```python
from build123d import *

# Parameters (mm, degrees)
SKETCH1_W            = 69
SKETCH1_H            = 165
BOSS_EXTRUDE1_DEPTH  = 7
SKETCH3_R            = 2.6
CUT_EXTRUDE2_DEPTH   = 7
SKETCH2_R            = 2.6
CUT_EXTRUDE1_DEPTH   = 7
SKETCH5_W            = 10
SKETCH5_H            = 10
BOSS_EXTRUDE2_DEPTH  = 23.264128691
SKETCH6_R            = 2.25
CUT_EXTRUDE3_DEPTH   = 10
FILLET1_R            = 10
FILLET1_OF_MIRROR1_R = 10
MIRROR2_START        = 123.910418582
MIRROR2_DEPTH        = 2.75
MIRROR2_START_2      = 116.660418582
MIRROR2_2_DEPTH      = 2.7499999
MIRROR2_START_3      = 119.410418482
MIRROR2_3_DEPTH      = 4.5000001
MIRROR2_START_4      = -23.264128691
MIRROR2_4_OUTLINE_R  = 2.25
MIRROR2_4_DEPTH      = 10


with BuildPart() as part:
    # Sketch1 → Boss-Extrude1 (new body)
    with BuildSketch(Plane.XY):
        with Locations((92.160418582, 14.328579343)):
            Rectangle(SKETCH1_W, SKETCH1_H)
    extrude(amount=BOSS_EXTRUDE1_DEPTH)

    # Sketch3 → Cut-Extrude2 (cut)
    with BuildSketch(Plane.XY.offset(7)):
        with Locations((109.883329943, 54.328579343)):
            Circle(SKETCH3_R)
        with Locations((109.883329943, -25.671420657)):
            Circle(SKETCH3_R)
    extrude(amount=-CUT_EXTRUDE2_DEPTH, mode=Mode.SUBTRACT)

    # Sketch2 → Cut-Extrude1 (cut)
    with BuildSketch(Plane.XY.offset(7)):
        with Locations((71.267526747, -59.671420657)):
            Circle(SKETCH2_R)
        with Locations((71.267526747, -15.671420657)):
            Circle(SKETCH2_R)
        with Locations((71.267526747, -7.671420657)):
            Circle(SKETCH2_R)
        with Locations((71.267526747, 36.328579343)):
            Circle(SKETCH2_R)
        with Locations((71.267526747, 44.328579343)):
            Circle(SKETCH2_R)
        with Locations((71.267526747, 88.328579343)):
            Circle(SKETCH2_R)
    extrude(amount=-CUT_EXTRUDE1_DEPTH, mode=Mode.SUBTRACT)

    # Sketch5 → Boss-Extrude2 (add)
    with BuildSketch(Plane(origin=(0, 0, 0), x_dir=(-1, 0, 0), z_dir=(0, 0, -1))):
        with Locations((-62.660418582, -63.171420657)):
            Rectangle(SKETCH5_W, SKETCH5_H)
    boss_extrude2 = extrude(amount=BOSS_EXTRUDE2_DEPTH)

    # Sketch6 → Cut-Extrude3 (cut)
    with BuildSketch(Plane(origin=(0, 0, -23.264128691), x_dir=(-1, 0, 0), z_dir=(0, 0, -1))):
        with Locations(Location((-62.660418582, -63.171420657, 0), (0, 0, 90))):
            Circle(SKETCH6_R)
    cut_extrude3 = extrude(amount=-CUT_EXTRUDE3_DEPTH, mode=Mode.SUBTRACT)

    # Fillet1
    fillet1_edges = [part.edges().sort_by_distance(p)[0] for p in [
        (62.660418582, -58.171420657, 0),
    ]]
    fillet(fillet1_edges, radius=FILLET1_R)

    # Mirror1: Boss-Extrude2, Cut-Extrude3 across plane
    add(boss_extrude2.mirror(Plane(origin=(0, 14.328579343, 0), x_dir=(0, 0, 1), z_dir=(0, -1, 0))))
    add(cut_extrude3.mirror(Plane(origin=(0, 14.328579343, 0), x_dir=(0, 0, 1), z_dir=(0, -1, 0))), mode=Mode.SUBTRACT)

    # Fillet1 of Mirror1
    fillet1_of_mirror1_edges = [part.edges().sort_by_distance(p)[0] for p in [
        (62.660418582, 86.828579343, 0),
    ]]
    fillet(fillet1_of_mirror1_edges, radius=FILLET1_OF_MIRROR1_R)

    # Mirror2: read off the stored shape, not the designer's step
    # Mirror2 outline → Mirror2 (add)
    with BuildSketch(Plane.YZ.offset(MIRROR2_START)):
        with BuildLine():
            ThreePointArc((-58.171420657, -10), (-55.242488469, -2.928932188), (-48.171420657, 0))
            Line((-48.171420657, 0), (-68.171420657, 0))
            Line((-68.171420657, 0), (-68.171420657, -23.264128691))
            Line((-68.171420657, -23.264128691), (-58.171420657, -23.264128691))
            Line((-58.171420657, -23.264128691), (-58.171420657, -10))
        make_face()
        with BuildLine():
            Line((96.828579343, -23.264128691), (96.828579343, 0))
            Line((96.828579343, 0), (76.828579343, 0))
            ThreePointArc((76.828579343, 0), (83.899647155, -2.928932188), (86.828579343, -10))
            Line((86.828579343, -10), (86.828579343, -23.264128691))
            Line((86.828579343, -23.264128691), (96.828579343, -23.264128691))
        make_face()
    extrude(amount=MIRROR2_DEPTH)

    # Mirror2 2 outline → Mirror2 2 (add)
    with BuildSketch(Plane.YZ.offset(MIRROR2_START_2)):
        with BuildLine():
            ThreePointArc((-58.171420657, -10), (-55.242488469, -2.928932188), (-48.171420657, 0))
            Line((-48.171420657, 0), (-68.171420657, 0))
            Line((-68.171420657, 0), (-68.171420657, -23.264128691))
            Line((-68.171420657, -23.264128691), (-58.171420657, -23.264128691))
            Line((-58.171420657, -23.264128691), (-58.171420657, -10))
        make_face()
        with BuildLine():
            Line((96.828579343, -23.264128691), (96.828579343, 0))
            Line((96.828579343, 0), (76.828579343, 0))
            ThreePointArc((76.828579343, 0), (83.899647155, -2.928932188), (86.828579343, -10))
            Line((86.828579343, -10), (86.828579343, -23.264128691))
            Line((86.828579343, -23.264128691), (96.828579343, -23.264128691))
        make_face()
    extrude(amount=MIRROR2_2_DEPTH)

    # Mirror2 3 outline → Mirror2 3 (add)
    with BuildSketch(Plane.YZ.offset(MIRROR2_START_3)):
        with BuildLine():
            Line((-68.171420657, -23.264128691), (-58.171420657, -23.264128691))
            Line((-58.171420657, -23.264128691), (-58.171420657, -10))
            ThreePointArc((-58.171420657, -10), (-55.242488469, -2.928932188), (-48.171420657, 0))
            Line((-48.171420657, 0), (-68.171420657, 0))
            Line((-68.171420657, 0), (-68.171420657, -23.264128691))
        make_face()
        with BuildLine():
            Line((96.828579343, 0), (76.828579343, 0))
            ThreePointArc((76.828579343, 0), (83.899647155, -2.928932188), (86.828579343, -10))
            Line((86.828579343, -10), (86.828579343, -23.264128691))
            Line((86.828579343, -23.264128691), (96.828579343, -23.264128691))
            Line((96.828579343, -23.264128691), (96.828579343, 0))
        make_face()
    extrude(amount=MIRROR2_3_DEPTH)

    # Mirror2 4 outline → Mirror2 4 (cut)
    with BuildSketch(Plane.XY.offset(MIRROR2_START_4)):
        with Locations((121.660418582, -63.171420657)):
            Circle(MIRROR2_4_OUTLINE_R)
        with Locations((121.660418582, 91.828579343)):
            Circle(MIRROR2_4_OUTLINE_R)
    extrude(amount=MIRROR2_4_DEPTH, mode=Mode.SUBTRACT)


solid = part.part
```
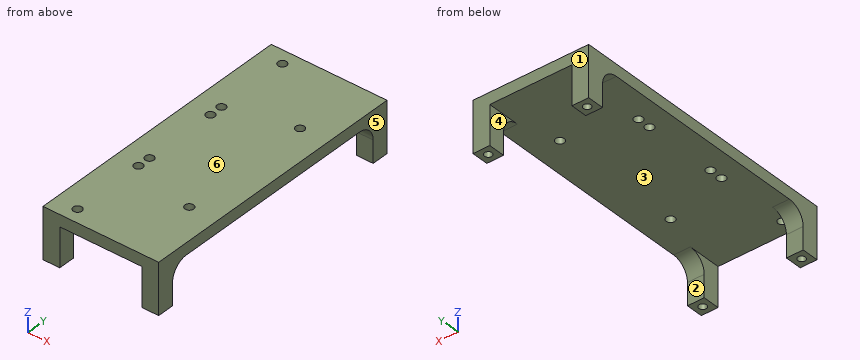
Source: CAD feature listing. Evaluate the final solid. Frame: model axes, mm. Face numbers are marked on the shaded views. A direction names the side the tool comes from. Round coordinates to 2 decimals unless told otherwise and drop trailing zeros. Loops run counter-clockwise (first coordinate to the right, second up) from the corner with the lowest first, then second, coordinate; pieces in that order, holes last.
1. Mould query, pull axis X, two halves, no side actions, for the marked faces 4, 5 and 6. Classes: released by +X, released by -X, zero draft, split by the parting line, or undercut.
2. Contact query for flat-ended pins moving along their axis: pin 1 (5 mm diameter, centred on x = 113.5, z = -6.5, fed in from -Y); pin 2 (8 mm diameter, centred on x = 81.5, y = -38.5, fed in from -Z). Output: stop coordinate, or through.
3. Section query B-B on y = -39. Output: boundary loops of the cut face in (x, z).
4. Ray query, L1, parallel to Y at x = 65.5, z = -19.5; L2, parallel to Z at x = 89.5, y = -29.5; L3, parallel to X at y = -58.5, z = -10. Return the intervals inside material, ascending.
5. Section query C-C on x = 77. Output: boundary loops of the cut face in (y, z).
6. Access query for the marked faces 1, 2 and 3. Directions: +Z, -Z, +X, -X, +Y, -Y. A direction counts if a zero-diameter tool reaches every point of the face in a straight line with its end or side. Return the directions, or none.
7. Section query A-A on z = -18.5. Output: boundary loops of the cut face in (x, y), and give its area (3 significant figures).
Answers below:
1. face 4: undercut
1. face 5: released by +X
1. face 6: zero draft
2. pin 1: passes through
2. pin 2: stops at z = 0
3. outline: (57.66, 0) - (126.66, 0) - (126.66, 7) - (57.66, 7) - close
4. L1: y = -68.17 to -58.17, 86.83 to 96.83
4. L2: z = 0 to 7
4. L3: x = 57.66 to 67.66, 116.66 to 126.66
5. outline: (-68.17, 0) - (96.83, 0) - (96.83, 7) - (-68.17, 7) - close
6. face 1: +Z, -Z, +X, -X, +Y
6. face 2: -Z, +X, -X
6. face 3: -Z
7. outline: (57.66, -68.17) - (67.66, -68.17) - (67.66, -58.17) - (57.66, -58.17) - close; (57.66, 86.83) - (67.66, 86.83) - (67.66, 96.83) - (57.66, 96.83) - close; (116.66, -68.17) - (126.66, -68.17) - (126.66, -58.17) - (116.66, -58.17) - close; (116.66, 86.83) - (126.66, 86.83) - (126.66, 96.83) - (116.66, 96.83) - close; hole circle Ø4.5 at (62.66, -63.17); hole circle Ø4.5 at (62.66, 91.83); hole circle Ø4.5 at (121.66, -63.17); hole circle Ø4.5 at (121.66, 91.83)
7. area: 336 mm2
